CAD build for the part. Positions are in the model's coordinates, mm. A direction names the side the tool comes from. Round coordinates to 2 decimals unless told otherwise and drop trailing zeros. Order: outer loops, then holes, each group sorted by start corner. A loop starts at its lowest first (then second) coordinate and runs counter-clockwise, first axis right, second up. Notation, with made-up numbers: (6.25, 33) - (59.25, 33) arc R28 cw to (59.25, 68) - close; hole circle Ø3 at (67.25, 5). An arc over 180 degrees is marked (long way). Use one line per item in the form item = value. Start each with the question number.
from build123d import *

# Parameters (mm, degrees)
ESBO_O1_W                = 91
ESBO_O1_H                = 63
ESBO_O1_W_2              = 87
ESBO_O1_H_2              = 59
RESSALTO_EXTRUS_O1_DEPTH = 5
ESBO_O2_W                = 91
ESBO_O2_H                = 63
RESSALTO_EXTRUS_O2_DEPTH = 2
FILETE6_R                = 1
FILETE7_R                = 1
FILETE10_R               = 1
FILETE11_R               = 1
FILETE12_R               = 1


with BuildPart() as part:
    # Esboço1 → Ressalto-extrusão1 (new body)
    with BuildSketch(Plane.XY):
        with Locations((-1.263340114, -15.201421801)):
            Rectangle(ESBO_O1_W, ESBO_O1_H)
        with Locations((-1.263340114, -15.201421801)):
            Rectangle(ESBO_O1_W_2, ESBO_O1_H_2, mode=Mode.SUBTRACT)
    extrude(amount=RESSALTO_EXTRUS_O1_DEPTH)

    # Esboço2 → Ressalto-extrusão2 (add)
    with BuildSketch(Plane(origin=(0, 0, 0), x_dir=(-1, 0, 0), z_dir=(0, 0, -1))):
        with Locations((1.263340114, -15.201421801)):
            Rectangle(ESBO_O2_W, ESBO_O2_H)
    extrude(amount=RESSALTO_EXTRUS_O2_DEPTH)

    # Filete6
    filete6_edges = [part.edges().sort_by_distance(p)[0] for p in [
        (42.236659886, 14.298578199, 2.5),
    ]]
    fillet(filete6_edges, radius=FILETE6_R)

    # Filete7
    filete7_edges = [part.edges().sort_by_distance(p)[0] for p in [
        (-44.763340114, 14.298578199, 2.5),
        (-44.763340114, -44.701421801, 2.5),
        (42.236659886, -44.701421801, 2.5),
    ]]
    fillet(filete7_edges, radius=FILETE7_R)

    # Filete10
    filete10_edges = [part.edges().sort_by_distance(p)[0] for p in [
        (-46.763340114, -46.701421801, 1.5),
    ]]
    fillet(filete10_edges, radius=FILETE10_R)

    # Filete11
    filete11_edges = [part.edges().sort_by_distance(p)[0] for p in [
        (-46.763340114, 16.298578199, 1.5),
        (44.236659886, 16.298578199, 1.5),
        (44.236659886, -46.701421801, 1.5),
    ]]
    fillet(filete11_edges, radius=FILETE11_R)

    # Filete12
    filete12_edges = [part.edges().sort_by_distance(p)[0] for p in [
        (-46.763340114, -15.201421801, -2),
        (-46.470446895, -46.408528582, -2),
        (44.236659886, -15.201421801, -2),
        (-1.263340114, -46.701421801, -2),
        (-1.263340114, 16.298578199, -2),
        (-46.470446895, 16.00568498, -2),
        (43.943766667, 16.00568498, -2),
        (43.943766667, -46.408528582, -2),
    ]]
    fillet(filete12_edges, radius=FILETE12_R)


solid = part.part
(1) Slice it at B-B (y = -5). Give the cut face in (x, z), and give its area (3 significant figures).
(2) Wall check: line 1 (Y direction, x = 3.5, z = 2); line 2 (X direction, y = 3, z = 2.75); line 3 (X direction, y = 13.5, z = 3). Give the ranges that are in metal, low to high. Write a range as [from, to].
(3) Which spindle directions (+Z, -Z, +X, -X, +Y, -Y) get a long thin tool onto all of the face, cutting with end or side? Do faces 5 (the flat face through (-44.763, -16, 2)), 6 (the flat face through (-5, -45, 5)). Say none if no direction does.
(4) Slice it at A-A (z = 2). Give the cut face in (x, y).
(5) Mould opens along X. For faces 1 (the flat face through (-1, -15, -2)), 2 (the flat face through (-46.763, -16, 2)), 3 (the flat face through (44.237, -16, 2)), 4 (the flat face through (-2, 14.299, 2)) say: pulls with the +X half, pulls with the -X half, needs draft (parallel to the pull), parting line crosses it, or undercut.
(6) Slice it at C-C (x = -18.5). Give the cut face in (y, z).
Results list:
q1.outline = (-46.76, -1) arc R1 ccw to (-45.76, -2) - (43.24, -2) arc R1 ccw to (44.24, -1) - (44.24, 5) - (42.24, 5) - (42.24, 0) - (-44.76, 0) - (-44.76, 5) - (-46.76, 5) - close
q1.area = 202 mm²
q2.line_1 = [-46.7, -44.7], [14.3, 16.3]
q2.line_2 = [-46.76, -44.76], [42.24, 44.24]
q2.line_3 = [-46.76, -44.74], [42.22, 44.24]
q3.face_5 = +Z
q3.face_6 = +Z, +X, -X, +Y, -Y
q4.outline = (-46.76, -45.7) arc R1 ccw to (-45.76, -46.7) - (43.24, -46.7) arc R1 ccw to (44.24, -45.7) - (44.24, 15.3) arc R1 ccw to (43.24, 16.3) - (-45.76, 16.3) arc R1 ccw to (-46.76, 15.3) - close; hole (-44.76, -43.7) arc R1 ccw to (-43.76, -44.7) - (41.24, -44.7) arc R1 ccw to (42.24, -43.7) - (42.24, 13.3) arc R1 ccw to (41.24, 14.3) - (-43.76, 14.3) arc R1 ccw to (-44.76, 13.3) - close
q5.face_1 = needs draft
q5.face_2 = pulls with the -X half
q5.face_3 = pulls with the +X half
q5.face_4 = undercut
q6.outline = (-46.7, -1) arc R1 ccw to (-45.7, -2) - (15.3, -2) arc R1 ccw to (16.3, -1) - (16.3, 5) - (14.3, 5) - (14.3, 0) - (-44.7, 0) - (-44.7, 5) - (-46.7, 5) - close
